```python
from build123d import *

# Parameters (mm, degrees)
BOSS_EXTRUDE1_DEPTH = 15
SKETCH5_R           = 6.25
CUT_EXTRUDE1_DEPTH  = 22
SKETCH7_W           = 20
SKETCH7_H           = 35
BOSS_EXTRUDE4_DEPTH = 48
SKETCH19_W          = 10
SKETCH19_H          = 20
CUT_EXTRUDE2_DEPTH  = 65
SKETCH22_W          = 60
SKETCH22_H          = 35
BOSS_EXTRUDE5_DEPTH = 12
SKETCH23_W          = 60
SKETCH23_H          = 8
BOSS_EXTRUDE6_DEPTH = 13


with BuildPart() as part:
    # Sketch3 → Boss-Extrude1 (new body)
    with BuildSketch(Plane(origin=(0, 0, 0), x_dir=(1, 0, 0), z_dir=(0, 1, 0))):
        with BuildLine():
            Line((-29.495428398, 31.401945846), (32.504571602, 31.401945846))
            ThreePointArc((32.504571602, 31.401945846), (37.100765679, 29.498139924), (39.004571602, 24.901945846))
            Line((39.004571602, 24.901945846), (39.004571602, -22.098054154))
            ThreePointArc((39.004571602, -22.098054154), (37.100765679, -26.694248232), (32.504571602, -28.598054154))
            Line((32.504571602, -28.598054154), (-29.495428398, -28.598054154))
            ThreePointArc((-29.495428398, -28.598054154), (-34.091622476, -26.694248232), (-35.995428398, -22.098054154))
            Line((-35.995428398, -22.098054154), (-35.995428398, 24.901945846))
            ThreePointArc((-35.995428398, 24.901945846), (-34.091622476, 29.498139924), (-29.495428398, 31.401945846))
        make_face()
    extrude(amount=BOSS_EXTRUDE1_DEPTH)

    # Sketch5 → Cut-Extrude1 (cut)
    with BuildSketch(Plane(origin=(0, 15, 0), x_dir=(1, 0, 0), z_dir=(0, 1, 0))):
        with Locations(Location((-22.5, -12.598054154, 0), (0, 0, 270))):
            Circle(SKETCH5_R)
        with Locations(Location((22.5, -12.598054154, 0), (0, 0, 270))):
            Circle(SKETCH5_R)
    extrude(amount=-CUT_EXTRUDE1_DEPTH, mode=Mode.SUBTRACT)

    # Sketch7 → Boss-Extrude4 (add, along a direction that is not the sketch's normal)
    with BuildSketch(Plane(origin=(0, 15, 0), x_dir=(1, 0, 0), z_dir=(0, 1, 0))):
        with Locations((-1.909590385, 13.901945846)):
            Rectangle(SKETCH7_W, SKETCH7_H)
    extrude(amount=BOSS_EXTRUDE4_DEPTH, dir=(0, 0.5000000000000001, -0.8660254037844387))

    # Sketch19 → Cut-Extrude2 (cut, along a direction that is not the sketch's normal)
    with BuildSketch(Plane(origin=(0, 12.808003151, 7.394704067), x_dir=(1, 0, 0), z_dir=(0, 0.8660254037844377, 0.5000000000000016))):
        with Locations((-1.909590385, 26.383993698)):
            Rectangle(SKETCH19_W, SKETCH19_H)
    extrude(amount=-CUT_EXTRUDE2_DEPTH, dir=(0, 1, 0), mode=Mode.SUBTRACT)

    # Sketch22 → Boss-Extrude5 (add)
    with BuildSketch(Plane(origin=(0, 39, 0), x_dir=(1, 0, 0), z_dir=(0, 1, 0))):
        with Locations((-1.909590385, 55.471165228)):
            Rectangle(SKETCH22_W, SKETCH22_H)
    extrude(amount=BOSS_EXTRUDE5_DEPTH)

    # Sketch23 → Boss-Extrude6 (add)
    with BuildSketch(Plane(origin=(0, 51, 0), x_dir=(1, 0, 0), z_dir=(0, 1, 0))):
        with Locations((-1.909590385, 41.971165228)):
            Rectangle(SKETCH23_W, SKETCH23_H)
    extrude(amount=BOSS_EXTRUDE6_DEPTH)


solid = part.part
```
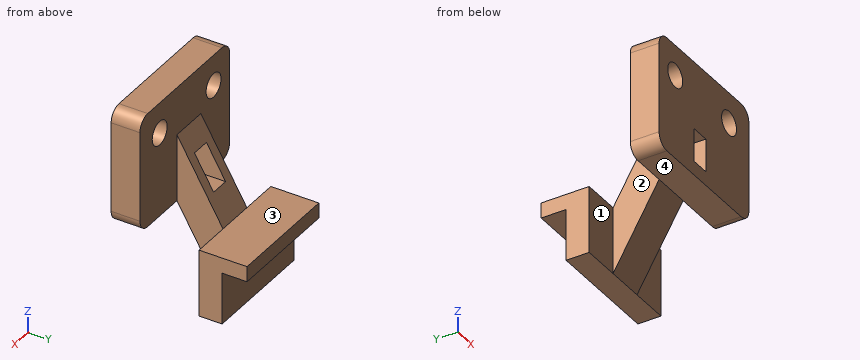
Design review of the part built by this model. Coordinates are the model's own, in mm. Face numbers are marked on the shaded views. A direction names the side the tool comes from. Round coordinates to 2 decimals unless told otherwise and drop trailing zeros. Write each loop counter-clockwise with the first axis right and the second up, starting at its lowest first coordinate (ties: lowest second). Pieces come first, ordered by that corner, then holes. Notation, with made-up numbers: (-3, 53) -> (45, 53) arc R19 ccw to (45, 57) -> close; hole circle Ø3 at (63, 22). An arc over 180 degrees is marked (long way). Write item = value, one per line. Start each with the question number.
1) Take a section at C-C, the plane z = -16.5. State the section outline as (x, y) points.
2) Clearance check with flat-ended pins moving along their axes: pin 1 (1.5 mm diameter, centred on x = -17.5, z = -56.5, fed in from -Y); pin 2 (1 mm diameter, centred on x = -21, z = -15.5, fed in from +Y); pin 3 (20 mm diameter, centred on x = 13, y = 57, fed in from +Z); pin 4 (14.5 mm diameter, centred on x = -5, y = 56, fed in from -Z). State where each tip first meets the part, or that it passes through.
3) Take a section at B-B, the plane x = -22.5. State the section outline as (y, z) points.
4) Take a section at D-D, the plane z = 10.5. State the section outline as (x, y) points, plus the area to 3 significant figures.
5) Tool access review of the marked faces 1, 2, 3 and 4: name each direction out of +Z, -Z, +X, -X, +Y, -Y from which nothing blocks a thin tool from reaching the whole face with its end or side.
6) Take a section at A-A, the plane x = 0. State the section outline as (y, z) points, plus the area to 3 significant figures.
7) Wall thickness on probe 1 along Z at (x, y) = (-23, 5.5); probe 2 along Z at (x, y) = (2, 4); probe 3 along Y at (x, z) = (-12.5, -49.5): over which ranges is each line inside the solid? List them lowest first. Write a range as from..to.
Results list:
q1.outline = (-36, 0) -> (-6.91, 0) -> (-6.91, 26.6) -> (-11.91, 26.6) -> (-11.91, 15) -> (-36, 15) -> close; (3.09, 0) -> (39, 0) -> (39, 15) -> (8.09, 15) -> (8.09, 26.6) -> (3.09, 26.6) -> close
q2.pin_1 = 39
q2.pin_2 = 15
q2.pin_3 = -37.97
q2.pin_4 = -72.97
q3.outline = (0, -31.4) -> (15, -31.4) -> (15, 6.35) -> (0, 6.35) -> close; (0, 18.85) -> (15, 18.85) -> (15, 28.6) -> (0, 28.6) -> close; (39, -72.97) -> (51, -72.97) -> (51, -45.97) -> (64, -45.97) -> (64, -37.97) -> (39, -37.97) -> close
q4.outline = (-36, 0) -> (-28.39, 0) -> (-28.39, 15) -> (-36, 15) -> close; (-16.61, 0) -> (16.61, 0) -> (16.61, 15) -> (-16.61, 15) -> close; (28.39, 0) -> (39, 0) -> (39, 15) -> (28.39, 15) -> close
q4.area = 772 mm²
q5.face_1 = +Z, -Z, -X, -Y
q5.face_2 = +Z, -Z, -X
q5.face_3 = +Z, +X, -X, +Y
q5.face_4 = -Z, +X, -X, -Y
q6.outline = (0, -31.4) -> (15, -31.4) -> (39, -72.97) -> (51, -72.97) -> (51, -45.97) -> (64, -45.97) -> (64, -37.97) -> (39, -37.97) -> (31, -24.11) -> (0, -24.11) -> close; (0, -6.79) -> (21, -6.79) -> (15, 3.6) -> (15, 28.6) -> (0, 28.6) -> close
q6.area = 1,810 mm²
q7.probe_1 = -31.4..6.37, 18.83..28.6
q7.probe_2 = -31.4..-24.11, -6.79..28.6
q7.probe_3 = 39..51
